The listing builds one solid part. Answer for the finished solid, in the listing's coordinates (mm). Face numbers are marked on the shaded views. Round coordinates to 2 decimals unless told otherwise and drop trailing zeros. Write each loop counter-clockwise with the first axis right and the second up, starting at its lowest first coordinate (ties: lowest second). Pieces come first, ordered by that corner, then holes. Notation, with made-up numbers: (16, -39) - (24, -39) arc R17 ccw to (24, -10) - close; hole circle Ø2 at (44.5, 87.25). An arc over 180 degrees is marked (long way). Return JSON: item names as keys, results as strings. Group by question number.
(1) Section B-B, the plane x = 0 is taken. Write down the section's boundary in (y, z).
(2) Each of these flat-tipped pins is pushed along its axis until it touches: pin 1 (12 mm diameter, centred on x = -17, z = -27, fed in from +Y); pin 2 (0.8 mm diameter, centred on x = -6, y = 0.5, fed in from -Z); pin 3 (5 mm diameter, centred on y = 2.5, z = -9.5, fed in from +X). Where does it stop, or does it pass through?
(3) Section A-A, the plane z = 0 is taken. Write down the section's boundary in (x, y).
(4) Find the intervals of material crossed by line 1 along X through (y, z) = (7, -2.5); line 2 along Z through (x, y) = (0, 18); line 3 along Y through (x, z) = (-64, 2.5), in increasing order. Write a range as [from, to].
(5) Section D-D, the plane x = -46.5 is taken. Write down the section's boundary in (y, z), then the cut area to 3 significant figures.
(6) Determine the mould class of the marked faces 1, 2, 3 and 4 for opening direction Z: +Z half, -Z half, draft (parallel to the pull), parting line (faces both ways), or undercut.
(7) Section C-C, the plane y = 17.75 is taken. Write down the section's boundary in (x, z), then the cut area to 3 significant figures.
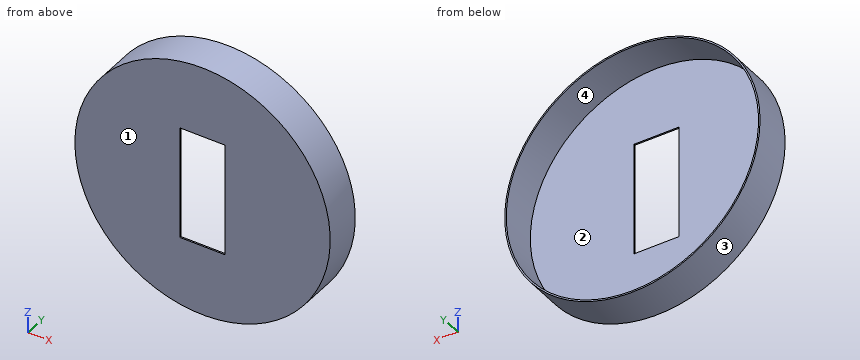
Autodesk Inventor part; units mm, degrees
ref_plane "YZ Plane" through (0, 0, 0) normal (1, 0, 0) x (0, 1, 0)
ref_plane "XZ Plane" through (0, 0, 0) normal (0, 1, 0) x (-1, 0, 0)
ref_plane "XY Plane" through (0, 0, 0) normal (0, 0, 1) x (1, 0, 0)
sketch "Sketch1" plane through (0, 0, 0) normal (0, 1, 0) x (-1, 0, 0)
  circle A0 centre (0, 0) radius 84.5
  line L0 (-15, 37.5) -> (15, 37.5)
  line L1 (15, 37.5) -> (15, -37.5)
  line L2 (15, -37.5) -> (-15, -37.5)
  line L3 (-15, -37.5) -> (-15, 37.5)
  line L4 (-15, 37.5) -> (15, -37.5) construction
  line L5 (15, 37.5) -> (-15, -37.5) construction
  dimension "d1" = 169
  dimension "d41" = 30
  dimension "d42" = 75
extrude "Extrusion4" add sketch "Sketch1" along normal blind 25.4
sketch "Sketch4" plane through (0, 25.4, 0) normal (0, 1, 0) x (1, 0, 0)
  circle A0 centre (0, 0) radius 83.5
  dimension "d45" = 167
hole "Hole2" at (0, 25.4, 0) direction (0, -1, 0) diameter 167 depth 24.4
ref_plane "Work Plane1" through (0, 0, 37.5) normal (1, 0, 0) x (0, 0, -1)
properties part number "Top Cap"
Working result:
{
 "1": {"outline": "(0, -84.5) - (25.4, -84.5) - (25.4, -83.5) - (1, -83.5) - (1, -37.5) - (0, -37.5) - close; (0, 37.5) - (1, 37.5) - (1, 83.5) - (25.4, 83.5) - (25.4, 84.5) - (0, 84.5) - close"},
 "2": {"pin 1": "stops at y = 1", "pin 2": "stops at z = -84.31", "pin 3": "stops at x = 84.21"},
 "3": {"outline": "(-84.5, 0) - (-15, 0) - (-15, 1) - (-83.5, 1) - (-83.5, 25.4) - (-84.5, 25.4) - close; (15, 0) - (84.5, 0) - (84.5, 25.4) - (83.5, 25.4) - (83.5, 1) - (15, 1) - close"},
 "4": {"line 1": "x = [-84.46, -83.46], [83.46, 84.46]", "line 2": "z = [-84.5, -83.5], [83.5, 84.5]", "line 3": "y = [0, 1]"},
 "5": {"outline": "(0, -70.55) - (25.4, -70.55) - (25.4, -69.35) - (1, -69.35) - (1, 69.35) - (25.4, 69.35) - (25.4, 70.55) - (0, 70.55) - close", "area": "200 mm^2"},
 "6": {"face 1": "draft", "face 2": "undercut", "face 3": "parting line", "face 4": "undercut"},
 "7": {"outline": "circle Ø169 at (0, 0); hole circle Ø167 at (0, 0)", "area": "528 mm^2"}
}
